Could you check a few things on this model? Use its own coordinates, in mm. Face numbers are marked on the shaded views. A direction names the side the tool comes from. Coordinates: 2 decimals unless noted, no trailing zeros. Write each loop counter-clockwise with the first axis right and the second up, starting at its lowest first coordinate (ties: lowest second). Pieces come first, ordered by that corner, then holes. Notation, with made-up numbers: (56, -5) - (74, -5) arc R29 cw to (74, 18) - close; hole circle Ø9 at (37, -37). An arc over 180 degrees is marked (long way). Answer as a JSON object with one key per item and string values. Group by question number.
1) Will these pins go through, and if not, where does the flat tip stop? pin 1 Ø1 at (x, y) = (45, 16) entering from -Z; pin 2 Ø1 at (x, y) = (44, 15.5) entering from +Z; pin 3 Ø8 at (x, z) = (-19.5, -8.5) entering from +Y.
2) On a 3-axis mill with a long thin cutter (end or side, diameter ignored), from which of +Z, -Z, +X, -X, +Y, -Y can I reach the whole of each face in a straight line? I mean the marked faces 1 and 2. Say none if no direction works.
3) If we section it at C-C (x = -2): Write out the boundary of the cut face in (y, z), plus the area to 3 significant figures.
4) If we section it at B-B (y = 5.75): Write out the boundary of the cut face in (x, z), plus the area to 3 significant figures.
5) If we section it at A-A (z = 31): Write out the boundary of the cut face in (x, y), plus the area to 3 significant figures.
6) Please list where these lines run through material, in increasing order: line 1 along Z through (x, y) = (-4, 22.25); line 2 along X through (y, z) = (22.25, -4.5); line 3 along Y through (x, z) = (44, 31).
7) We'd pull the mould along Z, two halves only. Please class the marked faces 3, 4 and 5: released by +Z, released by -Z, zero draft, split by the parting line, or undercut.
8) If we section it at D-D (z = -5.5): Write out the boundary of the cut face in (x, y), plus the area to 3 significant figures.
```python
from build123d import *

# Parameters (mm, degrees)
SKETCH_1_W               = 91
SKETCH_1_H               = 73
EXTRUDE_1_DEPTH          = 28
SKETCH_2_W               = 87
SKETCH_2_H               = 69
CUT_EXTRUDE_1_DEPTH      = 26
SKETCH_3_W               = 8
SKETCH_3_H               = 5
CUT_EXTRUDE_2_DEPTH      = 26
SKETCH_4_R               = 1.6
CUT_EXTRUDE_5_DEPTH      = 4
MIRROR_2_COPY_1_SKETCH_R = 1.6
MIRROR_2_COPY_1_DEPTH    = 4
FILLET_2_R               = 3
FILLET_3_R               = 3
FILLET_4_R               = 3
FILLET_5_R               = 3
FILLET_6_R               = 2
FILLET_7_R               = 2
FILLET_8_R               = 2
FILLET_9_R               = 2


with BuildPart() as part:
    # 草图1 → 凸台-拉伸1 (new body)
    with BuildSketch(Plane(origin=(0, 0, 0), x_dir=(1, 0, 0), z_dir=(0, 1, 0))):
        Rectangle(SKETCH_1_W, SKETCH_1_H)
    extrude(amount=EXTRUDE_1_DEPTH)

    # 草图2 → 切除-拉伸1 (cut)
    with BuildSketch(Plane(origin=(0, 28, 0), x_dir=(1, 0, 0), z_dir=(0, 1, 0))):
        Rectangle(SKETCH_2_W, SKETCH_2_H)
    extrude(amount=-CUT_EXTRUDE_1_DEPTH, mode=Mode.SUBTRACT)

    # 草图3 → 切除-拉伸2 (cut)
    with BuildSketch(Plane.ZY.offset(-43.5)):
        with Locations((-11.5, 16.5)):
            Rectangle(SKETCH_3_W, SKETCH_3_H)
    extrude(amount=-CUT_EXTRUDE_2_DEPTH, mode=Mode.SUBTRACT)

    # 草图4 → 切除-拉伸5 (cut)
    with BuildSketch(Plane.ZY.offset(-43.5)):
        with Locations((31, 23.4)):
            Circle(SKETCH_4_R)
    cut_extrude_5 = extrude(amount=-CUT_EXTRUDE_5_DEPTH, mode=Mode.SUBTRACT)

    # 镜向1: 切除-拉伸5 across plane
    add(cut_extrude_5.mirror(Plane.XY), mode=Mode.SUBTRACT)

    # 镜向2: 切除-拉伸5 across plane
    add(cut_extrude_5.mirror(Plane(origin=(0, 0, 0), x_dir=(0, 0, 1), z_dir=(1, 0, 0))), mode=Mode.SUBTRACT)

    # 镜向2 copy 1 sketch → 镜向2 copy 1 (cut)
    with BuildSketch(Plane(origin=(-43.5, 0, 0), x_dir=(0, 0, -1), z_dir=(1, 0, 0))):
        with Locations((31, 23.4)):
            Circle(MIRROR_2_COPY_1_SKETCH_R)
    extrude(amount=-MIRROR_2_COPY_1_DEPTH, mode=Mode.SUBTRACT)

    # 圆角2
    fillet_2_edges = [part.edges().sort_by_distance(p)[0] for p in [
        (45.5, 14, 36.5),
    ]]
    fillet(fillet_2_edges, radius=FILLET_2_R)

    # 圆角3
    fillet_3_edges = [part.edges().sort_by_distance(p)[0] for p in [
        (-45.5, 14, 36.5),
    ]]
    fillet(fillet_3_edges, radius=FILLET_3_R)

    # 圆角4
    fillet_4_edges = [part.edges().sort_by_distance(p)[0] for p in [
        (-45.5, 14, -36.5),
    ]]
    fillet(fillet_4_edges, radius=FILLET_4_R)

    # 圆角5
    fillet_5_edges = [part.edges().sort_by_distance(p)[0] for p in [
        (45.5, 14, -36.5),
    ]]
    fillet(fillet_5_edges, radius=FILLET_5_R)

    # 圆角6
    fillet_6_edges = [part.edges().sort_by_distance(p)[0] for p in [
        (-43.5, 15, -34.5),
    ]]
    fillet(fillet_6_edges, radius=FILLET_6_R)

    # 圆角7
    fillet_7_edges = [part.edges().sort_by_distance(p)[0] for p in [
        (43.5, 15, -34.5),
    ]]
    fillet(fillet_7_edges, radius=FILLET_7_R)

    # 圆角8
    fillet_8_edges = [part.edges().sort_by_distance(p)[0] for p in [
        (-43.5, 15, 34.5),
    ]]
    fillet(fillet_8_edges, radius=FILLET_8_R)

    # 圆角9
    fillet_9_edges = [part.edges().sort_by_distance(p)[0] for p in [
        (43.5, 15, 34.5),
    ]]
    fillet(fillet_9_edges, radius=FILLET_9_R)


solid = part.part
```
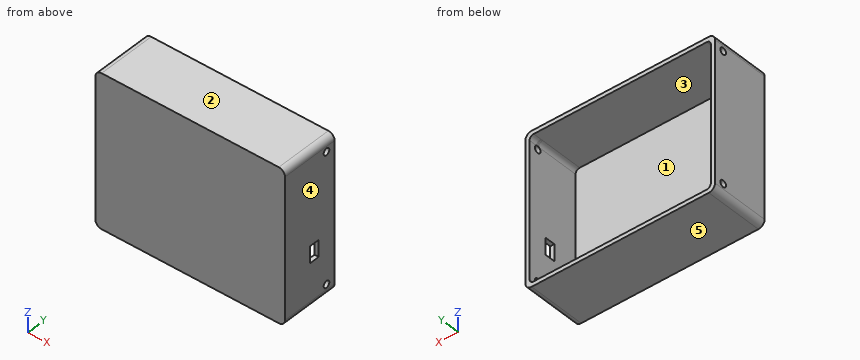
Here are the results:
{
 "1": {"pin 1": "stops at z = -35.74", "pin 2": "stops at z = 36.33", "pin 3": "stops at y = 2"},
 "2": {"face 1": "+Y", "face 2": "+Z, +X, -X, +Y, -Y"},
 "3": {"outline": "(0, -36.5) - (28, -36.5) - (28, -34.5) - (2, -34.5) - (2, 34.5) - (28, 34.5) - (28, 36.5) - (0, 36.5) - close", "area": "250 mm²"},
 "4": {"outline": "(-45.5, -33.5) arc R3 ccw to (-42.5, -36.5) - (42.5, -36.5) arc R3 ccw to (45.5, -33.5) - (45.5, 33.5) arc R3 ccw to (42.5, 36.5) - (-42.5, 36.5) arc R3 ccw to (-45.5, 33.5) - close; hole (-43.5, -32.5) arc R2 ccw to (-41.5, -34.5) - (41.5, -34.5) arc R2 ccw to (43.5, -32.5) - (43.5, 32.5) arc R2 ccw to (41.5, 34.5) - (-41.5, 34.5) arc R2 ccw to (-43.5, 32.5) - close", "area": "636 mm²"},
 "5": {"outline": "(-45.5, 0) - (45.5, 0) - (45.5, 21.8) - (43.5, 21.8) - (43.5, 2) - (-43.5, 2) - (-43.5, 21.8) - (-45.5, 21.8) - close; (-45.5, 25) - (-43.5, 25) - (-43.5, 28) - (-45.5, 28) - close; (43.5, 25) - (45.5, 25) - (45.5, 28) - (43.5, 28) - close", "area": "273 mm²"},
 "6": {"line 1": "z = -36.5 to -34.5, 34.5 to 36.5", "line 2": "x = -45.5 to -43.5, 43.5 to 45.5", "line 3": "y = 0 to 21.8, 25 to 28"},
 "7": {"face 3": "undercut", "face 4": "zero draft", "face 5": "released by -Z"},
 "8": {"outline": "(-45.5, 0) - (45.5, 0) - (45.5, 28) - (43.5, 28) - (43.5, 2) - (-43.5, 2) - (-43.5, 28) - (-45.5, 28) - close", "area": "286 mm²"}
}
